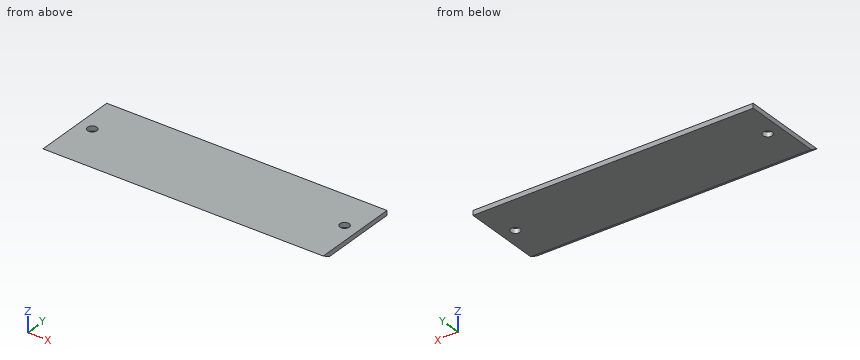
Autodesk Inventor part; units mm, degrees
ref_plane "YZ Plane" through (0, 0, 0) normal (1, 0, 0) x (0, 1, 0)
ref_plane "XZ Plane" through (0, 0, 0) normal (0, 1, 0) x (-1, 0, 0)
ref_plane "XY Plane" through (0, 0, 0) normal (0, 0, 1) x (1, 0, 0)
sketch "Szkic1" plane through (0, 0, 0) normal (0, 0, 1) x (1, 0, 0)
  line L0 (0, -19.6) -> (0, 19.6)
  line L1 (-63, 0) -> (63, 0)
  line L2 (-45, -14) -> (45, -14)
  line L3 (45, -14) -> (45, 14)
  line L4 (45, 14) -> (-45, 14)
  line L5 (-45, 14) -> (-45, -14)
  line L6 (-45, -14) -> (45, 14) construction
  line L7 (45, -14) -> (-45, 14) construction
  point P0 (0, 0)
  dimension "d0" = 28
  dimension "d1" = 90
extrude "Wyciągnięcie proste1" add sketch "Szkic1" along normal blind 1.5
sketch "Szkic3" plane through (45, -14, 0) normal (1, 0, 0) x (0, 0, -1)
  line L0 (-1.5, 0) -> (-1.5, 28)
  line L1 (0, 0) -> (0, 28)
  line L2 (0, 0) -> (0, 28)
  line L3 (0, 28) -> (-1.5, 28)
  line L4 (-1.5, 0) -> (-1.5, 28)
  line L5 (0, 0) -> (-1.5, 0)
  line L6 (-1.5, 0) -> (0, 2.5981)
  point P0 (0, 14)
  point P1 (0, 2.5981)
  dimension "d10" = 30
extrude "Wyciągnięcie proste3" cut sketch "Szkic3" against normal blind 100 contours L6 L1 L5
sketch "Szkic4" plane through (0, 0, 0) normal (0, 0, -1) x (-1, 0, 0)
  line L0 (-45, -11.4019) -> (-45, 14)
  line L1 (-45, 14) -> (45, 14)
  point P0 (0, 0)
  point P1 (-40.5, 1.5)
  dimension "d13" = 4.5
  dimension "d14" = 12.5
hole "Otwór1" at (40.5, 1.5, 0) direction (0, 0, 1) diameter 3 depth 4
mirror "Odbij1" about plane through (0, 0, 0) normal (1, 0, 0) of "Otwór1"
properties part number "pług_część1" material "Stal"
Geometry check sheet. Reference: the model listing, model coordinates, mm. Round coordinates to 2 decimals unless told otherwise and drop trailing zeros. Order: outer loops, then holes, each group sorted by start corner. A loop starts at its lowest first (then second) coordinate and runs counter-clockwise, first axis right, second up. Notation, with made-up numbers: (-18, -30) - (1, -30) arc R29 cw to (1, 7) - close; hole circle Ø3 at (28, 51.25). An arc over 180 degrees is marked (long way). One line per question, with ' | ' between items. Start each with the question number.
(1) Sectioned sample at A-A on y = 1.5. Record the cut outline in (x, z).
(2) Depth check by flat-ended pin: pin 1 Ø3.5 at (x, y) = (-40.5, 1.5) entering from -Z; pin 2 Ø2.5 at (x, y) = (40.5, 1.5) entering from +Z. Enter the tip coordinate at first touch or a pass-through.
(3) Sectioned sample at D-D on x = 18. Record the cut outline in (y, z), and give its area (3 significant figures).
(4) Sectioned sample at B-B on x = 40.5. Record the cut outline in (y, z), and give its area (3 significant figures).
(5) Thickness scan on L1, parallel to X at y = 1.5, z = 0.7; L2, parallel to Y at x = 40.5, z = 0.8; L3, parallel to Y at x = 40.5, z = 0.5. Record the ranges inside material, lowest first. Write a range as [from, to].
(6) Sectioned sample at C-C on z = 1. Record the cut outline in (x, y).
Conclusion:
1) outline: (-45, 0) - (-42, 0) - (-42, 1.5) - (-45, 1.5) - close; (-39, 0) - (39, 0) - (39, 1.5) - (-39, 1.5) - close; (42, 0) - (45, 0) - (45, 1.5) - (42, 1.5) - close
2) pin 1: stops at z = 0 | pin 2: passes through
3) outline: (-14, 1.5) - (-11.4, 0) - (14, 0) - (14, 1.5) - close | area: 40.1 mm2
4) outline: (-14, 1.5) - (-11.4, 0) - (0, 0) - (0, 1.5) - close; (3, 0) - (14, 0) - (14, 1.5) - (3, 1.5) - close | area: 35.6 mm2
5) L1: x = [-45, -42], [-39, 39], [42, 45] | L2: y = [-12.79, 0], [3, 14] | L3: y = [-12.27, 0], [3, 14]
6) outline: (-45, -13.13) - (45, -13.13) - (45, 14) - (-45, 14) - close; hole circle Ø3 at (-40.5, 1.5); hole circle Ø3 at (40.5, 1.5)
